Geometry: final body of the model. Coordinates: model frame, mm. A direction names the side the tool comes from. Give positions to 0.01 mm unless a question says otherwise; leave off trailing zeros. Write each loop counter-clockwise with the first axis right and the second up, starting at its lowest first coordinate (ties: lowest second). Pieces come first, ordered by that corner, then holes. Notation, with made-up numbers: M 22,-8.5 L 39,-8.5 A14 cw 39,4.5 Z; hole C -29.5,-24 d6. An arc over 180 degrees is marked long. Use a Markdown table: item, result. Add a question column.
(1) Draft query along Z for faces 3 (the cylindrical face through (-46.37, 14.79, -10.3)), 4 (the cylindrical face through (-43.48, 15.21, 0.29)), 5 (the flat face through (1, 30, 10)). Return one class per face: released by +Z, released by -Z, zero draft, split by the parting line, or undercut.
(2) Reachability of faces 1 (the flat face through (-7, 15, 0)), 2 (the cylindrical face through (0.676, 22.605, 27.146)) from +Z, -Z, +X, -X, +Y, -Y: full face, straight path, thin tool, end or side. Return the list, or none.
(3) Pin query (flat end, axial travel): pin 1 Ø2.5 at (x, z) = (-41.25, 0) entering from +Y; pin 2 Ø5 at (x, z) = (0, 25) entering from -Y; pin 3 Ø6 at (y, z) = (3, 18) entering from -X; pin 4 Ø6 at (x, z) = (0, -25) entering from +Y. Return the tip coordinate at first contact, or that it passes through.
(4) Cut plane B-B (z = 0). Output: boundary loops of the cut face in (x, y).
(5) Cut plane D-D (z = 25). Output: boundary loops of the cut face in (x, y).
(6) Cut plane A-A (x = 0). Output: boundary loops of the cut face in (y, z).
(7) Cut plane C-C (y = 7.75). Output: boundary loops of the cut face in (x, z), plus the area to 3 significant figures.
(8) Material intervals for L1, parallel to X at y = 14, z = 0; L2, parallel to X at y = 26.25, z = 0; L3, parallel to Z at x = -1, y = 4.25, sorted ascending.
```python
from build123d import *

# Parameters (mm, degrees)
SKETCH1_R           = 47.5
SKETCH1_R_2         = 35
BOSS_EXTRUDE1_DEPTH = 30
SKETCH2_R           = 2.25
CUT_EXTRUDE1_DEPTH  = 74.569694848
BOSS_EXTRUDE2_START = -15
SKETCH4_R           = 35
BOSS_EXTRUDE2_DEPTH = 15
SKETCH6_R           = 1.75
CUT_EXTRUDE2_DEPTH  = 30
SKETCH2_2_R         = 2.25
CUT_EXTRUDE3_DEPTH  = 74.569694848


with BuildPart() as part:
    # Sketch1 → Boss-Extrude1 (new body)
    with BuildSketch(Plane(origin=(0, 0, 0), x_dir=(1, 0, 0), z_dir=(0, 1, 0))):
        with Locations(Location((0, 0, 0), (0, 0, 270))):
            Circle(SKETCH1_R)
        with Locations(Location((0, 0, 0), (0, 0, 270))):
            Circle(SKETCH1_R_2, mode=Mode.SUBTRACT)
    extrude(amount=BOSS_EXTRUDE1_DEPTH)

    # Sketch2 → Cut-Extrude1 (cut, through all)
    with BuildSketch(Plane(origin=(0, 30, 0), x_dir=(1, 0, 0), z_dir=(0, 1, 0))):
        with Locations(Location((0, 41.25, 0), (0, 0, 270))):
            Circle(SKETCH2_R)
        with Locations(Location((41.25, 0, 0), (0, 0, 270))):
            Circle(SKETCH2_R)
        with Locations(Location((0, -41.25, 0), (0, 0, 90))):
            Circle(SKETCH2_R)
        with Locations(Location((-41.25, 0, 0), (0, 0, 90))):
            Circle(SKETCH2_R)
        with Locations((0, 25)):
            Circle(SKETCH2_R)
        with Locations((25, 0)):
            Circle(SKETCH2_R)
        with Locations((0, -25)):
            Circle(SKETCH2_R)
        with Locations((-25, 0)):
            Circle(SKETCH2_R)
    extrude(amount=-CUT_EXTRUDE1_DEPTH, mode=Mode.SUBTRACT)

    # Sketch4 → Boss-Extrude2 (add)
    with BuildSketch(Plane(origin=(0, 30, 0), x_dir=(1, 0, 0), z_dir=(0, 1, 0)).offset(BOSS_EXTRUDE2_START)):
        with Locations(Location((0, 0, 0), (0, 0, 270))):
            Circle(SKETCH4_R)
    extrude(amount=BOSS_EXTRUDE2_DEPTH)

    # Sketch6 → Cut-Extrude2 (cut)
    with BuildSketch(Plane(origin=(0, 30, 0), x_dir=(1, 0, 0), z_dir=(0, 1, 0))):
        with Locations(Location((0, 0, 0), (0, 0, 270))):
            Circle(SKETCH6_R)
    extrude(amount=-CUT_EXTRUDE2_DEPTH, mode=Mode.SUBTRACT)

    # Sketch2_2 → Cut-Extrude3 (cut, through all)
    with BuildSketch(Plane(origin=(0, 30, 0), x_dir=(1, 0, 0), z_dir=(0, 1, 0))):
        with Locations(Location((0, 41.25, 0), (0, 0, 270))):
            Circle(SKETCH2_2_R)
        with Locations(Location((41.25, 0, 0), (0, 0, 270))):
            Circle(SKETCH2_2_R)
        with Locations(Location((0, -41.25, 0), (0, 0, 90))):
            Circle(SKETCH2_2_R)
        with Locations(Location((-41.25, 0, 0), (0, 0, 90))):
            Circle(SKETCH2_2_R)
        with Locations(Location((0, 25, 0), (0, 0, 270))):
            Circle(SKETCH2_2_R)
        with Locations(Location((25, 0, 0), (0, 0, 270))):
            Circle(SKETCH2_2_R)
        with Locations(Location((0, -25, 0), (0, 0, 270))):
            Circle(SKETCH2_2_R)
        with Locations(Location((-25, 0, 0), (0, 0, 270))):
            Circle(SKETCH2_2_R)
    extrude(amount=-CUT_EXTRUDE3_DEPTH, mode=Mode.SUBTRACT)


solid = part.part
```
Answer list:
| question | item | result |
|---|---|---|
| 1 | face 3 | split by the parting line |
| 1 | face 4 | undercut |
| 1 | face 5 | zero draft |
| 2 | face 1 | -Y |
| 2 | face 2 | +Y, -Y |
| 3 | pin 1 | through |
| 3 | pin 2 | y = 15 |
| 3 | pin 3 | x = -45.07 |
| 3 | pin 4 | y = 30 |
| 4 | outline | M -47.5,0 L -43.5,0 L -43.5,30 L -47.5,30 Z; M -39,0 L -35,0 L -35,15 L -27.25,15 L -27.25,30 L -39,30 Z; M -22.75,15 L -1.75,15 L -1.75,30 L -22.75,30 Z; M 1.75,15 L 22.75,15 L 22.75,30 L 1.75,30 Z; M 27.25,15 L 35,15 L 35,0 L 39,0 L 39,30 L 27.25,30 Z; M 43.5,0 L 47.5,0 L 47.5,30 L 43.5,30 Z |
| 5 | outline | M -40.39,0 L -24.49,0 L -24.49,15 L -2.25,15 L -2.25,30 L -40.39,30 Z; M 2.25,15 L 24.49,15 L 24.49,0 L 40.39,0 L 40.39,30 L 2.25,30 Z |
| 6 | outline | M 0,-47.5 L 30,-47.5 L 30,-43.5 L 0,-43.5 Z; M 0,-39 L 30,-39 L 30,-27.25 L 15,-27.25 L 15,-35 L 0,-35 Z; M 0,35 L 15,35 L 15,27.25 L 30,27.25 L 30,39 L 0,39 Z; M 0,43.5 L 30,43.5 L 30,47.5 L 0,47.5 Z; M 15,-22.75 L 30,-22.75 L 30,-1.75 L 15,-1.75 Z; M 15,1.75 L 30,1.75 L 30,22.75 L 15,22.75 Z |
| 7 | outline | C 0,0 d95; hole C -41.25,0 d4.5; hole C 0,0 d70; hole C 0,-41.25 d4.5; hole C 0,41.25 d4.5; hole C 41.25,0 d4.5 |
| 7 | area | 3,180 mm² |
| 8 | L1 | -47.5 to -43.5, -39 to -35, 35 to 39, 43.5 to 47.5 |
| 8 | L2 | -47.5 to -43.5, -39 to -27.25, -22.75 to -1.75, 1.75 to 22.75, 27.25 to 39, 43.5 to 47.5 |
| 8 | L3 | -47.49 to -43.27, -39.23 to -34.99, 34.99 to 39.23, 43.27 to 47.49 |
